```python
from build123d import *

# Parameters (mm, degrees)
SKETCH1_W           = 42.3
SKETCH1_H           = 42.3
SKETCH1_R           = 1.5
BOSS_EXTRUDE1_DEPTH = 48
SKETCH2_R           = 11
BOSS_EXTRUDE2_DEPTH = 2
SKETCH3_R           = 2.5
BOSS_EXTRUDE3_DEPTH = 22
CHAMFER1_SIZE       = 4.5


with BuildPart() as part:
    # Sketch1 → Boss-Extrude1 (new body)
    with BuildSketch(Plane.XY):
        Rectangle(SKETCH1_W, SKETCH1_H)
        with Locations((-15.5, 15.5)):
            Circle(SKETCH1_R, mode=Mode.SUBTRACT)
        with Locations((15.5, 15.5)):
            Circle(SKETCH1_R, mode=Mode.SUBTRACT)
        with Locations((-15.5, -15.5)):
            Circle(SKETCH1_R, mode=Mode.SUBTRACT)
        with Locations((15.5, -15.5)):
            Circle(SKETCH1_R, mode=Mode.SUBTRACT)
    extrude(amount=BOSS_EXTRUDE1_DEPTH)

    # Sketch2 → Boss-Extrude2 (add)
    with BuildSketch(Plane.XY.offset(48)):
        Circle(SKETCH2_R)
    extrude(amount=BOSS_EXTRUDE2_DEPTH)

    # Sketch3 → Boss-Extrude3 (add)
    with BuildSketch(Plane.XY.offset(50)):
        Circle(SKETCH3_R)
    extrude(amount=BOSS_EXTRUDE3_DEPTH)

    # Chamfer1
    chamfer1_edges = [part.edges().sort_by_distance(p)[0] for p in [
        (-21.15, 21.15, 24),
        (21.15, 21.15, 24),
        (21.15, -21.15, 24),
        (-21.15, -21.15, 24),
    ]]
    chamfer(chamfer1_edges, length=CHAMFER1_SIZE)


solid = part.part
```
Could you check a few things on this model? Use its own coordinates, in mm. A direction names the side the tool comes from. Round coordinates to 2 decimals unless told otherwise and drop trailing zeros. Order: outer loops, then holes, each group sorted by start corner. A loop starts at its lowest first (then second) coordinate and runs counter-clockwise, first axis right, second up. Notation, with made-up numbers: M -24.75,41.5 L 34.25,41.5 A28 cw 34.25,60.5 Z; hole C 54.25,0.25 d4. An arc over 180 degrees is marked long. One line per question, with ' | ' between items. Start each with the question number.
(1) For P1, Ø2.5, axis at x = -15.5, y = 15.5, coming from the +Z side; P2, Ø3, axis at x = 8, y = -15.5, coming from the +Z side; P3, Ø6, axis at y = 2, z = 58.5, coming from the -X side; P4, Ø5, axis at x = 11, y = -2, coming from the +Z side, each with a flat end and sliding along its axis, tell me the tip position at first contact or that it passes through.
(2) For faces 4 (the face through (-2.38, -10.74, 48.99)), 5 (the face through (-17, 15.57, 23.66)), which set-ups out of +Z, -Z, +X, -X, +Y, -Y let a thin tool reach every point of the face, with its end or its side?
(3) Please list where these lines run through material, in increasing order: line 1 along Y through (x, z) = (15.5, 16.5); line 2 along X through (y, z) = (-15, 33).
(4) Suppose I cut it at D-D on x = 0. List the corners of the cut face in (y, z) for me.
(5) Suppose I cut it at A-A on y = -15.5. List the corners of the cut face in (x, z) for me, then the cut area to 3 significant figures.
(6) Thinking about a two-plate mould opening in Y: for faces 1 (the face through (-18.9, -18.9, 23.7)), 2 (the face through (14, -15.43, 23.66)), 3 (the face through (-3, 0, 50)), which applies, +Y half, -Y half, draft (parallel to the pull), parting line (faces both ways), or undercut?
(7) Suppose I cut it at C-C on z = 11. List the corners of the cut face in (x, y) for me.
Geometry results:
1) P1: through | P2: z = 48 | P3: x = -2.5 | P4: z = 50
2) face 4: +Z | face 5: +Z, -Z
3) line 1: -21.15 to -17, -14 to 14, 17 to 21.15 | line 2: -21.15 to -16.91, -14.09 to 14.09, 16.91 to 21.15
4) outline: M -21.15,0 L 21.15,0 L 21.15,48 L 11,48 L 11,50 L 2.5,50 L 2.5,72 L -2.5,72 L -2.5,50 L -11,50 L -11,48 L -21.15,48 Z
5) outline: M -21.15,0 L -17,0 L -17,48 L -21.15,48 Z; M -14,0 L 14,0 L 14,48 L -14,48 Z; M 17,0 L 21.15,0 L 21.15,48 L 17,48 Z | area: 1,740 mm²
6) face 1: -Y half | face 2: undercut | face 3: draft
7) outline: M -21.15,-16.65 L -16.65,-21.15 L 16.65,-21.15 L 21.15,-16.65 L 21.15,16.65 L 16.65,21.15 L -16.65,21.15 L -21.15,16.65 Z; hole C -15.5,-15.5 d3; hole C -15.5,15.5 d3; hole C 15.5,-15.5 d3; hole C 15.5,15.5 d3
